Input: part model. Units: mm. Frame: model coordinates. A direction names the side the tool comes from. Coordinates: 2 decimals unless noted, no trailing zeros. Loops run counter-clockwise (first coordinate to the right, second up) from the corner with the lowest first, then second, coordinate; pieces in that order, holes last.
```python
from build123d import *

# Parameters (mm, degrees)
SKETCH1_W            = 6.266
SKETCH1_H            = 19.6
SKETCH1_R            = 1.475
SKETCH1_W_2          = 52.832
SKETCH1_H_2          = 5
BOSS_EXTRUDE2_DEPTH  = 3.175
SKETCH3_W            = 30
SKETCH3_H            = 29.6
BOSS_EXTRUDE3_DEPTH  = 3.175
SKETCH4_R            = 4.75
CUT_EXTRUDE1_DEPTH   = 10
BOSS_EXTRUDE14_DEPTH = 3.175
CUT_EXTRUDE8_DEPTH   = 10
BOSS_EXTRUDE15_DEPTH = 3.175
BOSS_EXTRUDE16_DEPTH = 3.175
BOSS_EXTRUDE17_DEPTH = 3.175
FILLET5_R            = 4
SKETCH27_W           = 3.175
SKETCH27_H           = 8
CUT_EXTRUDE9_DEPTH   = 10
SKETCH28_W           = 18
SKETCH28_H           = 3.175
BOSS_EXTRUDE18_DEPTH = 3.175


with BuildPart() as part:
    # Sketch1 → Boss-Extrude2 (new body)
    # profile 1 of 4: a face of its own
    with BuildSketch(Plane.XY):
        with Locations((-23.283, 0)):
            Rectangle(SKETCH1_W, SKETCH1_H)
        with Locations((-23.95, -4.974)):
            Circle(SKETCH1_R, mode=Mode.SUBTRACT)
        with Locations((-23.95, 4.974)):
            Circle(SKETCH1_R, mode=Mode.SUBTRACT)
    # profile 2 of 4: a face of its own
    with BuildSketch(Plane.XY):
        with Locations((23.283, 0)):
            Rectangle(SKETCH1_W, SKETCH1_H)
        with Locations((23.95, -4.974)):
            Circle(SKETCH1_R, mode=Mode.SUBTRACT)
        with Locations((23.95, 4.974)):
            Circle(SKETCH1_R, mode=Mode.SUBTRACT)
    # profile 3 of 4: a face of its own
    with BuildSketch(Plane.XY):
        with Locations((0, 12.3)):
            Rectangle(SKETCH1_W_2, SKETCH1_H_2)
    # profile 4 of 4: a face of its own
    with BuildSketch(Plane.XY):
        with Locations((0, -12.3)):
            Rectangle(SKETCH1_W_2, SKETCH1_H_2)
    extrude(amount=BOSS_EXTRUDE2_DEPTH)

    # Sketch3 → Boss-Extrude3 (add)
    with BuildSketch(Plane.XY.offset(3.175)):
        with Locations((41.416, 0)):
            Rectangle(SKETCH3_W, SKETCH3_H)
    extrude(amount=-BOSS_EXTRUDE3_DEPTH)

    # Sketch4 → Cut-Extrude1 (cut)
    with BuildSketch(Plane(origin=(0, 0, 0), x_dir=(-1, 0, 0), z_dir=(0, 0, -1))):
        with Locations((-40.576, 7.77)):
            Circle(SKETCH4_R)
    extrude(amount=-CUT_EXTRUDE1_DEPTH, mode=Mode.SUBTRACT)

    # Sketch22 → Boss-Extrude14 (add)
    with BuildSketch(Plane(origin=(0, 0, 0), x_dir=(-1, 0, 0), z_dir=(0, 0, -1))):
        with BuildLine():
            ThreePointArc((-34.680262133, 14.8), (-40.576, 16.945), (-46.471737867, 14.8))
            Line((-46.471737867, 14.8), (-34.680262133, 14.8))
        make_face()
    extrude(amount=-BOSS_EXTRUDE14_DEPTH)

    # Sketch23 → Cut-Extrude8 (cut)
    with BuildSketch(Plane(origin=(0, 0, 0), x_dir=(-1, 0, 0), z_dir=(0, 0, -1))):
        with BuildLine():
            Line((-49.751, -14.8), (-49.751, 7.77))
            ThreePointArc((-49.751, 7.77), (-48.890866804, 11.648609936), (-46.471737867, 14.8))
            Line((-46.471737867, 14.8), (-56.416, 14.8))
            Line((-56.416, 14.8), (-56.416, -14.8))
            Line((-56.416, -14.8), (-49.751, -14.8))
        make_face()
    extrude(amount=-CUT_EXTRUDE8_DEPTH, mode=Mode.SUBTRACT)

    # Sketch24 → Boss-Extrude15 (add)
    with BuildSketch(Plane(origin=(0, 0, 0), x_dir=(-1, 0, 0), z_dir=(0, 0, -1))):
        Polygon((30.425, 14.8), (26.416, 14.8), (26.416, -14.8), (27.751006616, -14.8), (30.425, -14.8), align=None)
    extrude(amount=-BOSS_EXTRUDE15_DEPTH)

    # Sketch25 → Boss-Extrude16 (add)
    with BuildSketch(Plane(origin=(0, 0, 0), x_dir=(-1, 0, 0), z_dir=(0, 0, -1))):
        Polygon((30.425, 14.8), (30.425, 9.8), (33.6, 9.8), (33.6, 1.8), (30.425, 1.8), (30.425, -1.8), (33.6, -1.8), (33.6, -9.8), (30.425, -9.8), (30.425, -14.8), (31.879074074, -14.8), (38.6, -14.8), (38.6, 14.8), align=None)
    extrude(amount=-BOSS_EXTRUDE16_DEPTH)

    # Sketch26 → Boss-Extrude17 (add)
    with BuildSketch(Plane(origin=(0, 0, 0), x_dir=(-1, 0, 0), z_dir=(0, 0, -1))):
        with BuildLine():
            ThreePointArc((-40.224226578, 16.938253948), (-37.274351652, 16.330358823), (-34.680262133, 14.8))
            Line((-34.680262133, 14.8), (38.6, 14.8))
            ThreePointArc((38.6, 14.8), (-0.807884867, 16.02500278), (-40.224226578, 16.938253948))
        make_face()
    extrude(amount=-BOSS_EXTRUDE17_DEPTH)

    # Fillet5
    fillet5_edges = [part.edges().sort_by_distance(p)[0] for p in [
        (-38.6, 14.8, 1.5875),
    ]]
    fillet(fillet5_edges, radius=FILLET5_R)

    # Sketch27 → Cut-Extrude9 (cut)
    with BuildSketch(Plane(origin=(0, 0, 0), x_dir=(-1, 0, 0), z_dir=(0, 0, -1))):
        with Locations((-43.1635, -5.8)):
            Rectangle(SKETCH27_W, SKETCH27_H)
    extrude(amount=-CUT_EXTRUDE9_DEPTH, mode=Mode.SUBTRACT)

    # Sketch28 → Boss-Extrude18 (add)
    with BuildSketch(Plane(origin=(0, 0, 0), x_dir=(-1, 0, 0), z_dir=(0, 0, -1))):
        with Locations((-40.751, -16.3875)):
            Rectangle(SKETCH28_W, SKETCH28_H)
        with Locations((-5.65, -16.3875)):
            Rectangle(SKETCH28_W, SKETCH28_H)
        with Locations((29.6, -16.3875)):
            Rectangle(SKETCH28_W, SKETCH28_H)
    extrude(amount=-BOSS_EXTRUDE18_DEPTH)


solid = part.part
```
Item 1: Section query B-B (x = -23.95). Output: boundary loops of the cut face in (y, z) (3 decimals), then the cut area to 3 significant figures.
Result:
outline: (-17.975, 0) - (-6.449, 0) - (-6.449, 3.175) - (-17.975, 3.175) - close; (-3.499, 0) - (3.499, 0) - (3.499, 3.175) - (-3.499, 3.175) - close; (6.449, 0) - (15.292, 0) - (15.292, 3.175) - (6.449, 3.175) - close
area: 86.9 mm2
Item 2: Reachability of faces 5 (the face through (14.65, -16, 2)), 6 (the face through (49.751, -5, 2)), 7 (the face through (-32, -1.8, 2)), 8 (the face through (2.215, 16.063, 1.565)), 9 (the face through (41, -17.975, 2)) from +Z, -Z, +X, -X, +Y, -Y: full face, straight path, thin tool, end or side. Return the list, or none.
Result:
face 5: +Z, -Z, -Y
face 6: +Z, -Z, +X, +Y, -Y
face 7: +Z, -Z
face 8: +Z, -Z, -X, +Y
face 9: +Z, -Z, +X, -X, -Y
Item 3: Mould query, pull axis X, two halves, no side actions, for faces 1 (the face through (-37.446, 13.747, 1.61)), 2 (the face through (24.74, -3.73, 1.57)), 3 (the face through (-22.543, -4.531, 1.565)), 4 (the face through (6, -17.975, 2)). Classes: +X half, -X half, draft (parallel to the pull), parting line (faces both ways), or undercut.
Result:
face 1: -X half
face 2: undercut
face 3: undercut
face 4: draft
Item 4: Section query C-C (x = 7). Output: boundary loops of the cut face in (y, z) (3 decimals).
Result:
outline: (-17.975, 0) - (-9.8, 0) - (-9.8, 3.175) - (-17.975, 3.175) - close; (9.8, 0) - (16.189, 0) - (16.189, 3.175) - (9.8, 3.175) - close
Item 5: Contact query for flat-ended pins moving along their axis: P1, Ø1.6, axis at x = 43.5, z = 2, coming from the +Y side; P2, Ø1.6, axis at x = -32, z = 2.5, coming from the +Y side; P3, Ø4, axis at x = -23.95, y = 4.974, coming from the +Z side (3 decimals); P4, Ø1, axis at x = 7.5, z = 1, coming from the +Y side. Output: stop coordinate, or through.
Result:
P1: stops at y = 16.7
P2: stops at y = 15.05
P3: stops at z = 3.175
P4: stops at y = 16.21
Item 6: Section query D-D (z = 1.15). Count the separate pieces of the cut face and the enclosed holes in it, then the cut area to 3 significant figures.
Result:
separate pieces: 1
enclosed holes: 9
area: 1,910 mm2
Item 7: Section query A-A (y = -9). Output: boundary loops of the cut face in (x, z) (3 decimals), then the cut area to 3 significant figures.
Result:
outline: (-38.6, 0) - (-33.6, 0) - (-33.6, 3.175) - (-38.6, 3.175) - close; (-30.425, 0) - (-20.15, 0) - (-20.15, 3.175) - (-30.425, 3.175) - close; (20.15, 0) - (41.576, 0) - (41.576, 3.175) - (20.15, 3.175) - close; (44.751, 0) - (49.751, 0) - (49.751, 3.175) - (44.751, 3.175) - close
area: 132 mm2
Item 8: Line query: L1, parallel to X at y = -2, z = 1.6 (3 decimals); L2, parallel to X at y = -1.5, z = 2.5; L3, parallel to X at y = 6.5, z = 0.4 (3 decimals). Output: solid intervals per line, ascending.
Result:
L1: x = -38.6 to -33.6, -30.425 to -20.15, 20.15 to 41.576, 44.751 to 49.751
L2: x = -38.6 to -20.15, 20.15 to 49.75
L3: x = -38.6 to -33.6, -30.425 to -20.15, 20.15 to 35.999, 45.153 to 49.751
